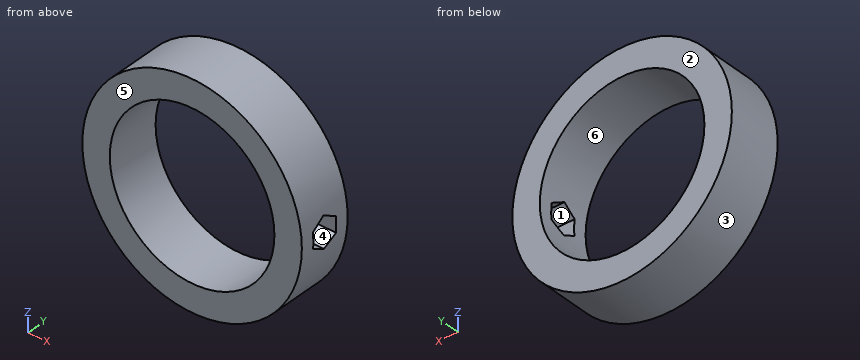
```python
from build123d import *

# Parameters (mm, degrees)
F0_R     = 40
F1_DEPTH = 10
F2_R     = 30
F3_DEPTH = 20
F5_DEPTH = 60


with BuildPart() as f1:
    # F0 (on Front) → F1 (new body, symmetric)
    with BuildSketch(Plane.XZ):
        Circle(F0_R)
    extrude(amount=F1_DEPTH, both=True)

    # F2 (on face) → F3 (cut, through all)
    with BuildSketch(Plane.XZ.offset(10)):
        Circle(F2_R)
    extrude(amount=-F3_DEPTH, mode=Mode.SUBTRACT)

    # F4 (on Right) → F5 (cut)
    with BuildSketch(Plane.YZ):
        Polygon((4.943565, 2.982364), (-0.111021, 5.772435), (-5.054586, 2.790071), (-4.943565, -2.982364), (0.111021, -5.772435), (5.054586, -2.790071), align=None)
    extrude(amount=F5_DEPTH, mode=Mode.SUBTRACT)


solid = f1.part
```
Work out the finished part from the listing and answer in its coordinate system (mm). Face numbers are marked on the shaded views. A direction names the side the tool comes from. Give positions to 0.01 mm unless a question says otherwise; leave off trailing zeros. Loops run counter-clockwise (first coordinate to the right, second up) from the corner with the lowest first, then second, coordinate; pieces in that order, holes last. Notation, with made-up numbers: (-34.5, 36.25) -> (15.5, 36.25) arc R17 ccw to (15.5, 41.25) -> close; hole circle Ø7 at (-8.75, 65.25). An arc over 180 degrees is marked (long way). Use CSV: the item, a comma, the result in double quotes.
1. The part is cut by section C-C (z = -20.5). Write down the section's boundary in (x, y), then the cut area to 3 significant figures.
Found:
outline,"(-34.35, -10) -> (-21.9, -10) -> (-21.9, 10) -> (-34.35, 10) -> close; (21.9, -10) -> (34.35, -10) -> (34.35, 10) -> (21.9, 10) -> close"
area,"498 mm^2"
2. Flat-ended cylindrical pins translate along their axes: pin 1 Ø4 at (x, y) = (-15.5, -1) entering from +Z; pin 2 Ø1 at (y, z) = (-6.5, -17) entering from +X; pin 3 Ø6 at (y, z) = (-1.5, -4.5) entering from -X. Find the tip coordinate at first contact, or state that the pin passes through.
Found:
pin 1,"z = 37.65"
pin 2,"x = 36.44"
pin 3,"x = -39.97"
3. Straight lines are drawn through the part: line 1 (Z direction, x = 0, y = -5.5); line 2 (X direction, y = -9, z = 1); line 3 (Z direction, x = 10.5, y = 1). For each, find the intervals that lie inside material, in ascending order.
Found:
line 1,"-40 to -30, 30 to 40"
line 2,"-39.99 to -29.98, 29.98 to 39.99"
line 3,"-38.6 to -28.1, 28.1 to 38.6"
4. The part is cut by section D-D (y = -7.75). Write down the section's boundary in (x, z), then the cut area to 3 significant figures.
Found:
outline,"circle Ø80 at (0, 0); hole circle Ø60 at (0, 0)"
area,"2,200 mm^2"
5. The part is cut by section B-B (z = 0). Write down the section's boundary in (x, y).
Found:
outline,"(-40, -10) -> (-30, -10) -> (-30, 10) -> (-40, 10) -> close; (30, -10) -> (40, -10) -> (40, -5) -> (30, -5) -> close; (30, 5) -> (40, 5) -> (40, 10) -> (30, 10) -> close"
6. The part is cut by section A-A (x = 0). Write down the section's boundary in (y, z).
Found:
outline,"(-10, -40) -> (10, -40) -> (10, -30) -> (-10, -30) -> close; (-10, 30) -> (10, 30) -> (10, 40) -> (-10, 40) -> close"
7. A tool of negligible diameter and unlimited length cuts with its end or side. For the marked faces 1 and 2, from which of +Z, -Z, +X, -X, +Y, -Y can it reach the whole face along a straight path? Write none if from no direction.
Found:
face 1,"+X"
face 2,"+Z, -Z, +X, -X, +Y"
8. The mould has two halves that part along Z. Classify the marked faces 3, 4, 5 and 6: +Z half, -Z half, draft (parallel to the pull), parting line (faces both ways), or undercut.
Found:
face 3,"parting line"
face 4,"undercut"
face 5,"draft"
face 6,"undercut"
